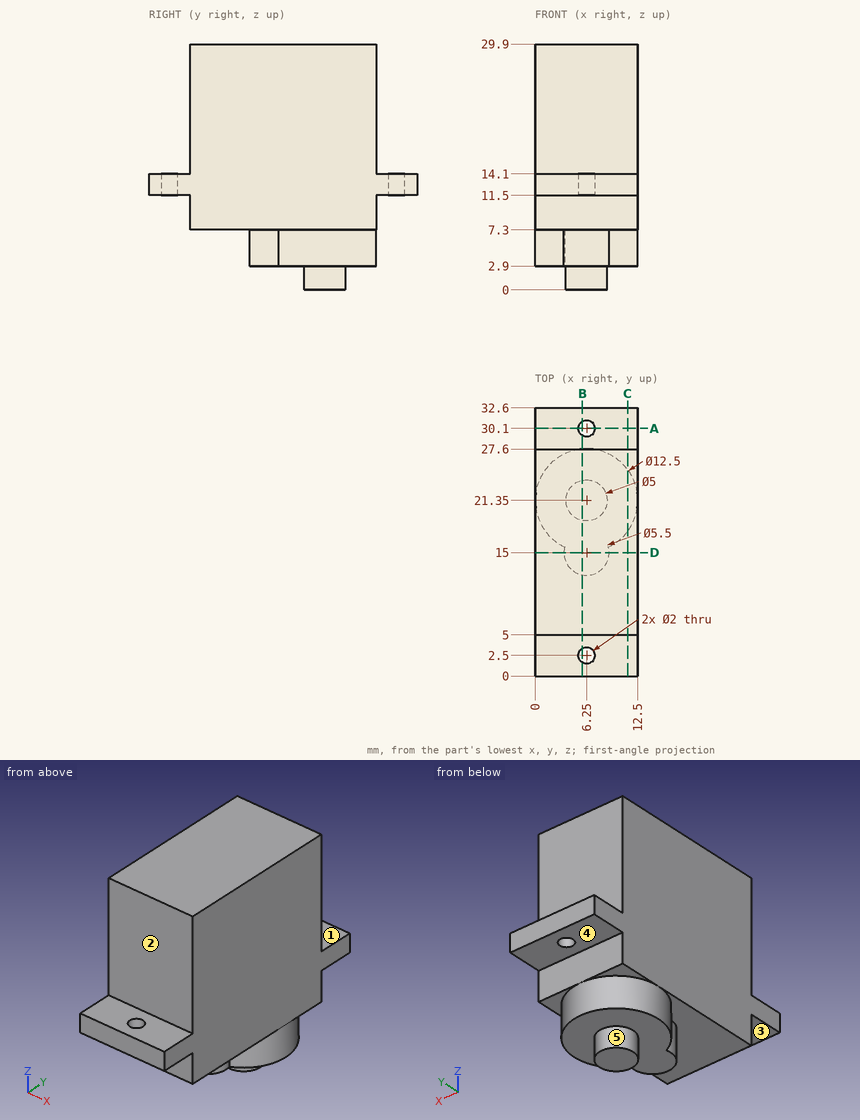
Verification items for this drawing (mm, ordinates from the low corner). A direction names the side the tool comes from. Give positions to 0.01 mm unless a question says otherwise; leave off trailing zeros. Write each loop counter-clockwise with the first axis right and the second up, starting at its lowest first coordinate (ties: lowest second). Pieces come first, ordered by that corner, then holes. Notation, with made-up numbers: (54.25, -36.75) - (87.25, -36.75) arc R21 cw to (87.25, -26.75) - close; hole circle Ø2 at (39, -13). An arc over 180 degrees is marked (long way). Answer as CSV lines item,"result". Start each with the question number.
1. Depth check by flat-ended pin: pin 1 (4 mm diameter, centred on x = 3.5, y = 31, fed in from +Z); pin 2 (4 mm diameter, centred on x = 8.5, z = 5, fed in from -Y); pin 3 (3 mm diameter, centred on x = 9.5, y = 24, fed in from -Z); pin 4 (6.5 mm diameter, centred on x = 5, y = 18.5, fed in from -Z). Enter the tip coordinate at first touch or a pass-through.
2. Sectioned sample at B-B (x = 5.75). Count the separate pieces of the cut face and the enclosed holes in it, then the cut area to 3 significant figures.
3. Sectioned sample at D-D (y = 15). Record the boundary of the cut face in (x, z).
4. Set-up check for the marked faces 1, 2, 3, 4 and 5: record each of +Z, -Z, +X, -X, +Y, -Y from which the full face is reachable in a straight line by a thin tool's end or side.
5. Sectioned sample at C-C (x = 11.25). Record the boundary of the cut face in (y, z).
6. Sectioned sample at A-A (y = 30.1). Record the boundary of the cut face in (x, z).
7. Thickness scan on line 1 (X direction, y = 30.1, z = 13.15); line 2 (Z direction, x = 2.5, y = 10); line 3 (Z direction, x = 9.25, y = 26.5). Record the ranges inside material, lowest first.
Derived:
1,pin 1,"z = 14.1"
1,pin 2,"y = 12.26"
1,pin 3,"z = 2.9"
1,pin 4,"z = 0"
2,separate pieces,"3"
2,enclosed holes,"0"
2,area,"609 mm²"
3,outline,"(0, 7.3) - (3.5, 7.3) - (3.5, 2.9) - (9, 2.9) - (9, 7.3) - (12.5, 7.3) - (12.5, 29.9) - (0, 29.9) - close"
4,face 1,"+Z, +X, -X, +Y"
4,face 2,"+Z, +X, -X, -Y"
4,face 3,"-Z, +X, -X, -Y"
4,face 4,"-Z, +X, -X, +Y"
4,face 5,"-Z"
5,outline,"(0, 11.5) - (5, 11.5) - (5, 7.3) - (17.6, 7.3) - (17.6, 2.9) - (25.1, 2.9) - (25.1, 7.3) - (27.6, 7.3) - (27.6, 11.5) - (32.6, 11.5) - (32.6, 14.1) - (27.6, 14.1) - (27.6, 29.9) - (5, 29.9) - (5, 14.1) - (0, 14.1) - close"
6,outline,"(0, 11.5) - (5.25, 11.5) - (5.25, 14.1) - (0, 14.1) - close; (7.25, 11.5) - (12.5, 11.5) - (12.5, 14.1) - (7.25, 14.1) - close"
7,line 1,"0 to 5.25, 7.25 to 12.5"
7,line 2,"7.3 to 29.9"
7,line 3,"2.9 to 29.9"
